Source: CAD feature listing. Evaluate the final solid. Frame: model axes, mm. Round coordinates to 2 decimals unless told otherwise and drop trailing zeros.
```python
from build123d import *

# Parameters (mm, degrees)
CROQUIS1_W              = 300
CROQUIS1_H              = 50
CROQUIS1_R              = 7.5
SALIENTE_EXTRUIR1_DEPTH = 30
REDONDEO1_R             = 25
CROQUIS2_R              = 7.5
SALIENTE_EXTRUIR2_DEPTH = 15
REDONDEO2_R             = 5


with BuildPart() as part:
    # Croquis1 → Saliente-Extruir1 (new body)
    with BuildSketch(Plane.XY):
        with Locations((150, 25)):
            Rectangle(CROQUIS1_W, CROQUIS1_H)
        with Locations((275, 25)):
            Circle(CROQUIS1_R, mode=Mode.SUBTRACT)
    extrude(amount=SALIENTE_EXTRUIR1_DEPTH)

    # Redondeo1
    redondeo1_edges = [part.edges().sort_by_distance(p)[0] for p in [
        (300, 0, 15),
        (300, 50, 15),
    ]]
    fillet(redondeo1_edges, radius=REDONDEO1_R - 0.0001)  # a hair under: the kernel refuses the full size

    # Croquis2 → Saliente-Extruir2 (add)
    with BuildSketch(Plane.ZY):
        with Locations((15, 25)):
            Circle(CROQUIS2_R)
    extrude(amount=SALIENTE_EXTRUIR2_DEPTH)

    # Redondeo2
    redondeo2_edges = [part.edges().sort_by_distance(p)[0] for p in [
        (137.50005, 50, 0),
        (292.677698819, 42.677698819, 0),
        (292.677698819, 7.322301181, 0),
        (137.50005, 50, 30),
        (292.677698819, 42.677698819, 30),
        (292.677698819, 7.322301181, 30),
        (0, 25, 30),
        (137.50005, 0, 0),
        (0, 25, 0),
        (137.50005, 0, 30),
        (0, 50, 15),
        (0, 0, 15),
    ]]
    fillet(redondeo2_edges, radius=REDONDEO2_R)


solid = part.part
```
Q1. Line query: line 1 (Y direction, x = 275, z = 12.75); line 2 (Y direction, x = 218.5, z = 4.5); line 3 (X direction, y = 2, z = 18). Output: solid intervals per line, ascending.
Q2. Mould query, pull axis Y, two halves, no side actions, for faces 1 (the face through (1, 25, 28)), 2 (the face through (281.93, 22.13, 14.79)), 3 (the face through (142, 48, 1)). Classes: pulls with the +Y half, pulls with the -Y half, needs draft (parallel to the pull), parting line crosses it, or undercut.
Q3. Pin query (flat end, axial travel): P1, Ø8, axis at y = 39.5, z = 23, coming from the +X side; P2, Ø12, axis at x = 275, y = 25, coming from the -Z side. Return the tip coordinate at first contact, or that it passes through.
Filled in:
1. line 1: y = 0 to 17.5, 32.5 to 50
1. line 2: y = 0.03 to 49.97
1. line 3: x = 1 to 284.8
2. face 1: needs draft
2. face 2: undercut
2. face 3: pulls with the +Y half
3. P1: stops at x = 297.69
3. P2: passes through
